from build123d import *

# Parameters (mm, degrees)
ESQUISSE1_W             = 42.5
ESQUISSE1_H             = 28
BOSS_EXTRU_1_DEPTH      = 3
ESQUISSE2_R             = 1.25
ENL_V_MAT_EXTRU_1_DEPTH = 3
ESQUISSE3_W             = 13.5
ESQUISSE3_H             = 28
BOSS_EXTRU_2_DEPTH      = 13
ESQUISSE4_W             = 12
ESQUISSE4_H             = 23.4
ENL_V_MAT_EXTRU_2_DEPTH = 43.355637169
CONG_1_R                = 0.5
CONG_2_R                = 1


with BuildPart() as part:
    # Esquisse1 → Boss.-Extru.1 (new body)
    with BuildSketch(Plane.XY):
        with Locations((-21.25, -14)):
            Rectangle(ESQUISSE1_W, ESQUISSE1_H)
    extrude(amount=BOSS_EXTRU_1_DEPTH)

    # Esquisse2 → Enlèv. mat.-Extru.1 (cut)
    with BuildSketch(Plane(origin=(0, 0, 0), x_dir=(-1, 0, 0), z_dir=(0, 0, -1))):
        with Locations((39.25, -24.75)):
            Circle(ESQUISSE2_R)
        with Locations((26.75, -24.75)):
            Circle(ESQUISSE2_R)
        with Locations(Location((39.25, -3.25, 0), (0, 0, 180))):
            Circle(ESQUISSE2_R)
        with Locations(Location((26.75, -3.25, 0), (0, 0, 180))):
            Circle(ESQUISSE2_R)
    extrude(amount=-ENL_V_MAT_EXTRU_1_DEPTH, mode=Mode.SUBTRACT)

    # Esquisse3 → Boss.-Extru.2 (add)
    with BuildSketch(Plane(origin=(0, 0, 0), x_dir=(-1, 0, 0), z_dir=(0, 0, -1))):
        with Locations((6.75, -14)):
            Rectangle(ESQUISSE3_W, ESQUISSE3_H)
    extrude(amount=BOSS_EXTRU_2_DEPTH)

    # Esquisse4 → Enlèv. mat.-Extru.2 (cut, through all)
    with BuildSketch(Plane.ZY.offset(13.5)):
        with Locations((-6, -14)):
            Rectangle(ESQUISSE4_W, ESQUISSE4_H)
    extrude(amount=-ENL_V_MAT_EXTRU_2_DEPTH, mode=Mode.SUBTRACT)

    # Congé1
    cong_1_edges = [part.edges().sort_by_distance(p)[0] for p in [
        (-6.75, -25.7, -12),
        (-6.75, -2.3, -12),
        (-6.75, -2.3, 0),
        (-6.75, -25.7, 0),
    ]]
    fillet(cong_1_edges, radius=CONG_1_R)

    # Congé2
    cong_2_edges = [part.edges().sort_by_distance(p)[0] for p in [
        (-6.75, -28, -13),
        (-6.75, 0, -13),
    ]]
    fillet(cong_2_edges, radius=CONG_2_R)


solid = part.part
The listing builds one solid part. Answer for the finished solid, in the listing's coordinates (mm). A direction names the side the tool comes from. Round coordinates to 2 decimals unless told otherwise and drop trailing zeros. Loops run counter-clockwise (first coordinate to the right, second up) from the corner with the lowest first, then second, coordinate; pieces in that order, holes last. Notation, with made-up numbers: M 7.5,-16 L 66.5,-16 A22 cw 66.5,10 Z; hole C 23,71 d4. An arc over 180 degrees is marked long. Write each question's results on one line, items separated by ' | '. Start each with the question number.
1) Find section A-A on x = -26.75. Write down the section's boundary in (y, z), plus the area to 3 significant figures.
2) Find section C-C on y = -18.5. Write down the section's boundary in (x, z), plus the area to 3 significant figures.
3) Determine the mould class of faces 4 (the cylindrical face through (-25.595, -2.771, 1.479)), 5 (the flat face through (0, -14.2, 0.4)), 6 (the flat face through (-7, -25.7, -6)) for opening direction X: pulls with the +X half, pulls with the -X half, needs draft (parallel to the pull), parting line crosses it, or undercut.
4) Which of the six approach directions +Z, -Z, +X, -X, +Y, -Y give full straight-line access (tool end or side, diameter ignored) to faces 1 (the flat face through (-22, -14, 0)), 2 (the flat face through (-7, -2.3, -6)), 3 (the flat face through (-13.5, -14.1, -12.2))?
5) Straight lines are drawn through the part: probe 1 along Y at (x, z) = (-26.75, 0.6); probe 2 along X at (y, z) = (-3.25, 2); probe 3 along Y at (x, z) = (-2, -6.75). For each, find the intervals that lie inside material, in ascending order.
6) Find section B-B on z = -5. Write down the section's boundary in (x, y), plus the area to 3 significant figures.
7) Each of these flat-tipped pins is pushed along its axis until it touches: pin 1 (5 mm diameter, centred on x = -22.5, y = -14, fed in from -Z); pin 2 (2 mm diameter, centred on x = -26.75, y = -24.75, fed in from -Z). Where does it stop, or does it pass through?
8) Find section D-D on z = 0.5. Write down the section's boundary in (x, y), plus the area to 3 significant figures.
Final values:
1) outline: M -28,0 L -26,0 L -26,3 L -28,3 Z; M -23.5,0 L -4.5,0 L -4.5,3 L -23.5,3 Z; M -2,0 L 0,0 L 0,3 L -2,3 Z | area: 69.0 mm²
2) outline: M -42.5,0 L 0,0 L 0,3 L -42.5,3 Z; M -13.5,-13 L 0,-13 L 0,-12 L -13.5,-12 Z | area: 141 mm²
3) face 4: undercut | face 5: pulls with the +X half | face 6: needs draft
4) face 1: -X | face 2: +X, -X | face 3: -Z, -X, +Y, -Y
5) probe 1: -28 to -26, -23.5 to -4.5, -2 to 0 | probe 2: -42.5 to -40.5, -38 to -28, -25.5 to 0 | probe 3: -28 to -25.7, -2.3 to 0
6) outline: M -13.5,-28 L 0,-28 L 0,-25.7 L -13.5,-25.7 Z; M -13.5,-2.3 L 0,-2.3 L 0,0 L -13.5,0 Z | area: 62.1 mm²
7) pin 1: z = 0 | pin 2: through
8) outline: M -42.5,-28 L 0,-28 L 0,0 L -42.5,0 Z; hole C -39.25,-24.75 d2.5; hole C -39.25,-3.25 d2.5; hole C -26.75,-24.75 d2.5; hole C -26.75,-3.25 d2.5 | area: 1,170 mm²
